from build123d import *

# Parameters (mm, degrees)
SKETCH1_R           = 10
SKETCH1_W           = 1200
SKETCH1_H           = 20
BOSS_EXTRUDE2_DEPTH = 20


with BuildPart() as part:
    # Sketch1 → Boss-Extrude2 (new body)
    with BuildSketch(Plane(origin=(0, 0, 0), x_dir=(1, 0, 0), z_dir=(0, 1, 0))):
        with Locations((-94.844294643, 267.550423494)):
            Circle(SKETCH1_R)
        with Locations((1105.155705357, 267.550423494)):
            Circle(SKETCH1_R)
        with Locations((305.155705357, -32.449576506)):
            Circle(SKETCH1_R)
        with Locations((705.155705357, -32.449576506)):
            Circle(SKETCH1_R)
        with BuildLine():
            Line((305.155705357, -22.449576506), (705.155705357, -22.449576506))
            Line((705.155705357, -22.449576506), (705.155705357, -42.449576506))
            Line((705.155705357, -42.449576506), (305.155705357, -42.449576506))
            ThreePointArc((305.155705357, -42.449576506), (315.155705357, -32.449576506), (305.155705357, -22.449576506))
        make_face()
        with Locations((505.155705357, 267.550423494)):
            Rectangle(SKETCH1_W, SKETCH1_H)
        Polygon((-88.844294643, 275.550423494), (311.155705357, -24.449576506), (302.050378198, -41.95520343), (-103.100204886, 261.907733883), align=None)
        Polygon((1113.4116156, 261.907733883), (711.164164437, -40.443225203), (699.147246278, -24.455927809), (1099.155705268, 275.550423427), align=None)
    extrude(amount=BOSS_EXTRUDE2_DEPTH)


solid = part.part
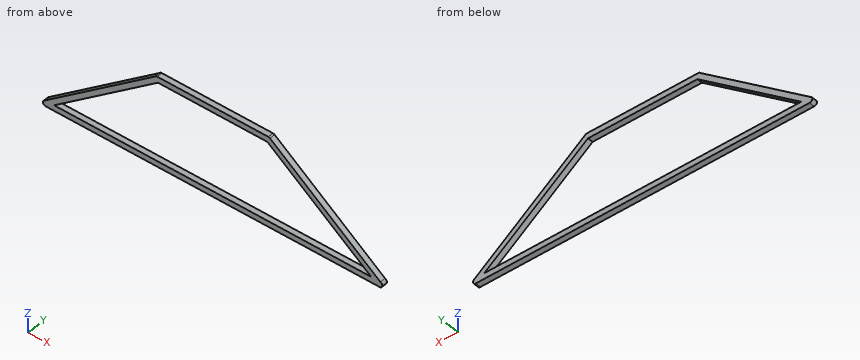
Verification items for the finished model (mm, model axes). Give positions to 0.01 mm unless a question says otherwise; leave off trailing zeros. Write each loop counter-clockwise with the first axis right and the second up, starting at its lowest first coordinate (ties: lowest second). Pieces come first, ordered by that corner, then holes. Notation, with made-up numbers: M 44,29 L 82,29 A18 ccw 82,47 Z; hole C 25,-28.5 d4. An arc over 180 degrees is marked long. Write item = value, one per line.
(1) Go/stop test with flat-tipped pins: pin 1 Ø1 at (x, y) = (856.5, 13) entering from +Z; pin 2 Ø5 at (y, z) = (14.5, -221) entering from -X; pin 3 Ø6 at (y, z) = (7, -65.5) entering from +X. Record where each tip stops, or that it passes through.
Found:
pin_1 = -68.42
pin_2 = -51.89
pin_3 = 856.1
(2) Sectioned sample at A-A (x = 555). Record the cut outline in (y, z).
Found:
outline = M 0,-277.55 L 20,-277.55 L 20,-257.55 L 0,-257.55 Z; M 0,22.45 L 20,22.45 L 20,42.45 L 0,42.45 Z
(3) Material ranges on line 1 (Z direction, x = 505.5, y = 19.25); line 2 (X direction, y = 7, z = -246.5); line 3 (Z direction, x = 138, y = 17.25), recorded low to high.
Found:
line_1 = -277.55 to -257.55, 22.45 to 42.45
line_2 = -82.56 to -50.11, 1060.42 to 1092.91
line_3 = -277.55 to -257.55, -105.42 to -81.08
(4) Sectioned sample at B-B (y = 17). Record the cut outline in (x, z), then the cut area to 3 significant figures.
Found:
outline = M -97.95,-258.04 A10 ccw -94.84,-277.55 L 1105.16,-277.55 A10 ccw 1108.28,-258.05 L 711.16,40.44 A10 ccw 705.16,42.45 L 305.16,42.45 A10 ccw 296.9,38.09 Z; hole M -64.84,-257.55 L 1075.16,-257.55 L 701.82,22.45 L 308.49,22.45 Z
area = 51,300 mm2
(5) Sectioned sample at C-C (z = -170.5). Record the cut outline in (x, y), then the cut area to 3 significant figures.
Found:
outline = M 18.78,0 L 51.22,0 L 51.22,20 L 18.78,20 Z; M 959.09,0 L 991.8,0 L 991.8,20 L 959.09,20 Z
area = 1,300 mm2
